Can you work these out from the drawing? Everything is in mm from the part's minimum corner. Give positions to 0.01 mm unless a question says otherwise; leave off trailing zeros. Loops run counter-clockwise (first coordinate to the right, second up) from the corner with the lowest first, then second, coordinate; pieces in that order, holes last. Notation, with made-up numbers: (24, 29.5) -> (44, 29.5) arc R22 ccw to (44, 52.5) -> close; hole circle Ø5 at (48.25, 3). An arc over 180 degrees is marked (long way). Return JSON: item names as keys, results as strings. Group by question number.
Q1. Thinking about a two-plate mould opening in Y: for the marked faces 1, 2 and 3, which applies, pulls with the +Y half, pulls with the -Y half, needs draft (parallel to the pull), parting line crosses it, or undercut?
Q2. Will these pins go through, and if not, where does the flat tip stop? pin 1 (1.5 mm diameter, centred on y = 0.5, z = 7, fed in from +X); pin 2 (1.5 mm diameter, centred on x = 4, z = 10, fed in from -Y); pin 3 (1.5 mm diameter, centred on x = 2, z = 8.5, fed in from +Y); pin 4 (2 mm diameter, centred on x = 3.5, y = 1.5, fed in from +Z).
Q3. Suppose I cut it at B-B, the plane x = 1.25. Please give me the cut outline in (y, z).
Q4. Suppose I cut it at A-A, the plane z = 12.25. Please give me the cut outline in (x, y).
Q5. Suppose I cut it at C-C, the plane y = 0.45. Please give me the cut outline in (x, z), and give its area (3 significant figures).
Q6. I need wall thicknesses on line 1 along X through (y, z) = (1.1, 13.5); line 2 along Z through (x, y) = (0.5, 0.25). Which ranges of each line are inside material? Lowest first, please. Write a range as [from, to].
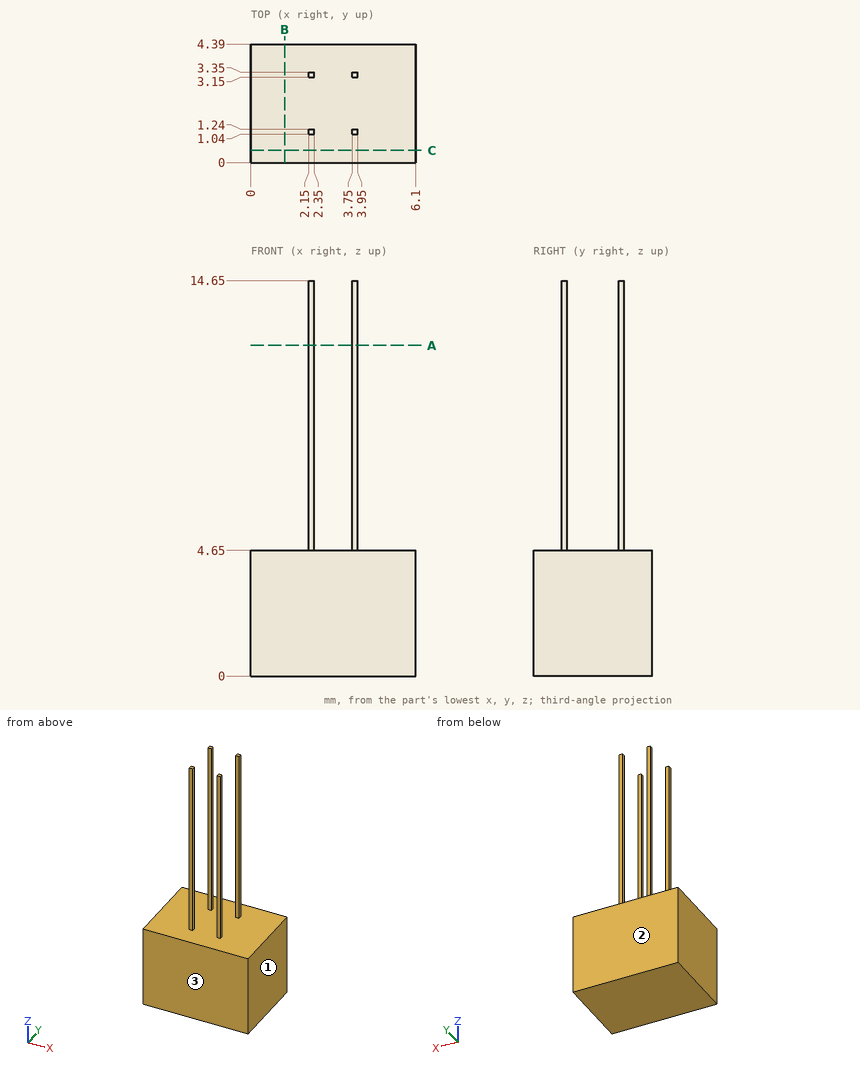
Ans:
{
 "1": {"face 1": "needs draft", "face 2": "pulls with the +Y half", "face 3": "pulls with the -Y half"},
 "2": {"pin 1": "stops at x = 3.95", "pin 2": "stops at y = 1.04", "pin 3": "stops at y = 3.35", "pin 4": "stops at z = 14.65"},
 "3": {"outline": "(0, 0) -> (4.39, 0) -> (4.39, 4.65) -> (0, 4.65) -> close"},
 "4": {"outline": "(2.15, 1.04) -> (2.35, 1.04) -> (2.35, 1.24) -> (2.15, 1.24) -> close; (2.15, 3.15) -> (2.35, 3.15) -> (2.35, 3.35) -> (2.15, 3.35) -> close; (3.75, 1.04) -> (3.95, 1.04) -> (3.95, 1.24) -> (3.75, 1.24) -> close; (3.75, 3.15) -> (3.95, 3.15) -> (3.95, 3.35) -> (3.75, 3.35) -> close"},
 "5": {"outline": "(0, 0) -> (6.1, 0) -> (6.1, 4.65) -> (0, 4.65) -> close", "area": "28.4 mm^2"},
 "6": {"line 1": "x = [2.15, 2.35], [3.75, 3.95]", "line 2": "z = [0, 4.65]"}
}
